Autodesk Inventor part; units mm, degrees
ref_plane "YZ Plane" through (0, 0, 0) normal (1, 0, 0) x (0, 1, 0)
ref_plane "XZ Plane" through (0, 0, 0) normal (0, 1, 0) x (-1, 0, 0)
ref_plane "XY Plane" through (0, 0, 0) normal (0, 0, 1) x (1, 0, 0)
sketch "Szkic1" plane through (0, 0, 0) normal (0, 0, 1) x (1, 0, 0)
  circle A0 centre (0, 0) radius 3.7
  circle A1 centre (0, 0) radius 2.575
  dimension "d0" = 7.4
  dimension "d1" = 5.15
extrude "Wyciągnięcie proste1" add sketch "Szkic1" along normal mid plane 25.3
chamfer "Faza1" distance 0.25 angle 45 2 edges at (-2.575, 0, 12.65) (-2.575, 0, -12.65)
properties part number "TULEJKA" material "Stal nierdzewna"
Can you work these out from the model? Positions are in its coordinate system, mm. Round coordinates to 2 decimals unless told otherwise and drop trailing zeros. Write each loop counter-clockwise with the first axis right and the second up, starting at its lowest first coordinate (ties: lowest second). Pieces come first, ordered by that corner, then holes. Notation, with made-up numbers: (76, 26) -> (87, 26) arc R15 ccw to (87, 34) -> close; hole circle Ø5 at (14, 64). An arc over 180 degrees is marked (long way). One line per question, with ' | ' between items. Start each with the question number.
1) I need wall thicknesses on line 1 (Y direction, x = 0, z = 5.5) (3 decimals); line 2 (X direction, y = -0.25, z = -11.25); line 3 (X direction, y = 1, z = 0.5). Which ranges of each line are inside material? Lowest first, please. Write a range as [from, to].
2) Suppose I cut it at C-C on z = -3. Write out the boundary of the cut face in (x, y) (3 decimals), then the cut area to 3 significant figures.
3) I'm going to push flat-ended pins straight in: P1, Ø1, axis at x = -1.5, z = 4, coming from the +Y side; P2, Ø3, axis at x = 1.5, y = 0.5, coming from the +Z side. Where does each tip first touch, or does it pass through?
4) If we mould it in two halves opening along X, with no side actions, what happens to faces 1 (the cylindrical face through (-0.802, -3.612, 0.177)), 2 (the cylindrical face through (2.456, -0.773, -0.174)), 3 (the flat face through (-1, -3, 12.65))? For each: released by +X, released by -X, zero draft, split by the parting line, or undercut.
5) Suppose I cut it at A-A on x = 0. Write out the boundary of the cut face in (y, z) (3 decimals), then the cut area to 3 significant figures.
Return value:
1) line 1: y = [-3.7, -2.575], [2.575, 3.7] | line 2: x = [-3.69, -2.56], [2.56, 3.69] | line 3: x = [-3.56, -2.37], [2.37, 3.56]
2) outline: circle Ø7.4 at (0, 0); hole circle Ø5.15 at (0, 0) | area: 22.2 mm2
3) P1: stops at y = 3.56 | P2: stops at z = 12.65
4) face 1: split by the parting line | face 2: undercut | face 3: zero draft
5) outline: (-3.7, -12.65) -> (-2.825, -12.65) -> (-2.575, -12.4) -> (-2.575, 12.4) -> (-2.825, 12.65) -> (-3.7, 12.65) -> close; (2.575, -12.4) -> (2.825, -12.65) -> (3.7, -12.65) -> (3.7, 12.65) -> (2.825, 12.65) -> (2.575, 12.4) -> close | area: 56.8 mm2
